Input: part model. Units: mm. Frame: model coordinates. A direction names the side the tool comes from. Round coordinates to 2 decimals unless told otherwise and drop trailing zeros. Order: outer loops, then holes, each group sorted by start corner. A loop starts at its lowest first (then second) coordinate and runs counter-clockwise, first axis right, second up. Notation, with made-up numbers: (17.25, 71) - (43.25, 71) arc R12 ccw to (43.25, 81) - close; hole circle Ø8 at (88.5, 75). An arc over 180 degrees is marked (long way). One line per item, written item: value. Start each with the question number.
Autodesk Inventor part; units mm, degrees
ref_plane "YZ Plane" through (0, 0, 0) normal (1, 0, 0) x (0, 1, 0)
ref_plane "XZ Plane" through (0, 0, 0) normal (0, 1, 0) x (-1, 0, 0)
ref_plane "XY Plane" through (0, 0, 0) normal (0, 0, 1) x (1, 0, 0)
sketch "Sketch1" plane through (0, 0, 0) normal (0, 0, 1) x (1, 0, 0)
  circle A0 centre (0, 0) radius 5.0674
  circle A1 centre (0, 0) radius 2.5
  circle A2 centre (0, 0) radius 7
  point P0 (0, 0)
  dimension "d0" = 5
  dimension "d1" = 14
extrude "Extrusion1" add sketch "Sketch1" along normal blind 5 contours A0 | A2
sketch "Sketch2" plane through (0, 0, 5) normal (0, 0, 1) x (1, 0, 0)
  circle A0 centre (0, 0) radius 2.5931
  circle A1 centre (0, 0) radius 2.5
  circle A2 centre (0, 0) radius 8
  dimension "d4" = 16
extrude "Extrusion2" add sketch "Sketch2" against normal blind 1 contours A2
chamfer "Chamfer1" distance 0.5 angle 45 1 edges at (-7, 0, 0)
properties part number "Flanged Bearing"
Item 1: Line query: L1, parallel to Y at x = 0, z = 2.15; L2, parallel to X at y = 1.75, z = 3.75; L3, parallel to Z at x = 3.75, y = 6. Output: solid intervals per line, ascending.
Item 2: First-contact query: pin 1 Ø3 at (x, z) = (-4.5, 3.5) entering from +Y; pin 2 Ø3 at (y, z) = (6, 1.5) entering from +X; pin 3 Ø1 at (y, z) = (1, 1.5) entering from -X; pin 4 Ø4.5 at (x, y) = (0, 0) entering from +Z. Flat tips, straight axial feed; report the tip coordinate or a pass-through.
Item 3: Section query C-C on z = 0.75. Return loops of the section in (x, y), and give its area (3 significant figures).
Item 4: Section query A-A on x = 0. Return loops of the section in (y, z).
Item 5: Pull-direction query (X, two-part tool) for faces 3 (the face through (4, -6, 4)), 4 (the face through (-1.73, -7.81, 4.51)), 5 (the face through (-0.54, 2.44, 2.46)); classes: released by +X, released by -X, zero draft, split by the parting line, or undercut.
Item 6: Reachability of faces 1 (the face through (-2, -2, 5)), 2 (the face through (6.466, 2.681, 2.226)) from +Z, -Z, +X, -X, +Y, -Y: full face, straight path, thin tool, end or side. Return the list, or none.
Geometry results:
1. L1: y = -7 to -2.5, 2.5 to 7
1. L2: x = -6.78 to -1.79, 1.79 to 6.78
1. L3: z = 4 to 5
2. pin 1: stops at y = 7.38
2. pin 2: stops at x = 5.36
2. pin 3: stops at x = -6.98
2. pin 4: passes through
3. outline: circle Ø14 at (0, 0); hole circle Ø5 at (0, 0)
3. area: 134 mm^2
4. outline: (-8, 4) - (-7, 4) - (-7, 0.5) - (-6.5, 0) - (-2.5, 0) - (-2.5, 5) - (-8, 5) - close; (2.5, 0) - (6.5, 0) - (7, 0.5) - (7, 4) - (8, 4) - (8, 5) - (2.5, 5) - close
5. face 3: zero draft
5. face 4: split by the parting line
5. face 5: undercut
6. face 1: +Z, +X, -X, +Y, -Y
6. face 2: -Z
